```python
from build123d import *

# Parameters (mm, degrees)
BOSS_EXTRUDE1_DEPTH      = 8.255
SKETCH2_R                = 4.52165068
CUT_EXTRUDE1_DEPTH       = 24.892
BOSS_EXTRUDE2_DEPTH      = 2.54
BOSS_EXTRUDE2_DEPTH_BACK = 19.05
BOSS_EXTRUDE3_DEPTH      = 55.87439679
SKETCH8_W                = 306.493093546
SKETCH8_H                = 19.05
BOSS_EXTRUDE4_DEPTH      = 55.87439679
SKETCH9_R                = 88.9
BOSS_EXTRUDE5_DEPTH      = 19.05
SKETCH10_W               = 191.766813877
SKETCH10_H               = 13.52799874
BOSS_EXTRUDE6_DEPTH      = 55.87439679
SKETCH12_R               = 1.75
CUT_EXTRUDE3_DEPTH       = 25.146
SKETCH14_R               = 12.700759967
CUT_EXTRUDE4_DEPTH       = 30.48
CUT_EXTRUDE5_DEPTH       = 55.118
SKETCH16_R               = 79.375
CUT_EXTRUDE6_DEPTH       = 16.129
CUT_EXTRUDE7_DEPTH       = 8.89
CUT_EXTRUDE8_DEPTH       = 2.54
SKETCH19_W               = 282.174011185
SKETCH19_H               = 80.01
CUT_EXTRUDE9_DEPTH       = 75.946
SKETCH20_R               = 79.375
BOSS_EXTRUDE7_DEPTH      = 19.05
SKETCH21_R               = 2.8
SKETCH21_R_2             = 2.794
CUT_EXTRUDE10_DEPTH      = 9.1
SKETCH22_R               = 79.375
CUT_EXTRUDE11_DEPTH      = 18.161
BOSS_EXTRUDE8_DEPTH      = 5.08
SKETCH24_R               = 80.01
CUT_EXTRUDE12_DEPTH      = 18.161


with BuildPart() as part:
    # Sketch1 → Boss-Extrude1 (new, symmetric)
    with BuildSketch(Plane(origin=(0, 0, 0), x_dir=(1, 0, 0), z_dir=(0, 1, 0))):
        Polygon((-26.685513069, 19.73834527), (-3.435840979, 33.16154971), (26.859514241, -19.311544765), (3.609842152, -32.734749204), align=None)
    extrude(amount=BOSS_EXTRUDE1_DEPTH, both=True)

    # Sketch2 → Cut-Extrude1 (cut)
    with BuildSketch(Plane(origin=(0, 8.255, 0), x_dir=(1, 0, 0), z_dir=(0, 1, 0))):
        with Locations(Location((0, 0, 0), (0, 0, 270))):
            Circle(SKETCH2_R)
    extrude(amount=-CUT_EXTRUDE1_DEPTH, mode=Mode.SUBTRACT)

    # Sketch12 → Cut-Extrude3 (cut)
    with BuildSketch(Plane(origin=(0, 8.255, 0), x_dir=(1, 0, 0), z_dir=(0, 1, 0))):
        with Locations(Location((-3.182842434, 15.553762143, 0), (0, 0, 270))):
            Circle(SKETCH12_R)
        with Locations(Location((3.182843419, -15.553761764, 0), (0, 0, 270))):
            Circle(SKETCH12_R)
        with Locations(Location((-11.87853102, 10.533303997, 0), (0, 0, 270))):
            Circle(SKETCH12_R)
        with Locations(Location((11.878532006, -10.533303617, 0), (0, 0, 270))):
            Circle(SKETCH12_R)
    extrude(amount=-CUT_EXTRUDE3_DEPTH, mode=Mode.SUBTRACT)


with BuildPart() as body_2:
    # Sketch3 → Boss-Extrude2 (new, two sides: drawn at the far end of the back side and taken through both)
    with BuildSketch(Plane(origin=(0, 8.255, 0), x_dir=(1, 0, 0), z_dir=(0, 1, 0)).offset(-BOSS_EXTRUDE2_DEPTH_BACK)):
        Polygon((-10.314271596, 73.739239236), (-58.702918637, 45.802040841), (10.314271596, -73.739239236), (58.702918637, -45.802040841), align=None)
        Polygon((-26.685513069, 19.73834527), (3.609842152, -32.734749204), (26.859514241, -19.311544765), (-3.435840979, 33.16154971), align=None, mode=Mode.SUBTRACT)
    extrude(amount=BOSS_EXTRUDE2_DEPTH + BOSS_EXTRUDE2_DEPTH_BACK)

    # Sketch7 → Boss-Extrude3 (add)
    with BuildSketch(Plane(origin=(-24.19432352, 0, 13.968599197), x_dir=(0.5000000000000003, 0, 0.8660254037844384), z_dir=(-0.8660254037844385, 0, 0.5000000000000004))):
        Polygon((-90.607190232, 10.795), (-118.92932164, -90.805), (-97.33932164, -90.805), (-69.017190232, -10.795), (-69.017190232, 10.795), align=None)
    boss_extrude3 = extrude(amount=-BOSS_EXTRUDE3_DEPTH)

    # Sketch8 → Boss-Extrude4 (add)
    with BuildSketch(Plane(origin=(-24.19432352, 0, 13.968599197), x_dir=(0.5000000000000003, 0, 0.8660254037844384), z_dir=(-0.8660254037844385, 0, 0.5000000000000004))):
        with Locations((0, -100.33)):
            Rectangle(SKETCH8_W, SKETCH8_H)
    extrude(amount=-BOSS_EXTRUDE4_DEPTH)

    # Mirror1: Boss-Extrude3 across plane
    add(boss_extrude3.mirror(Plane(origin=(-0.070654873, 0, -0.122377831), x_dir=(-0.8660254037844366, 0, 0.5000000000000038), z_dir=(0.5000000000000041, 0, 0.8660254037844364))))

    # Sketch9 → Boss-Extrude5 (add)
    with BuildSketch(Plane(origin=(0, -90.805, 0), x_dir=(1, 0, 0), z_dir=(0, 1, 0))):
        Circle(SKETCH9_R)
    extrude(amount=-BOSS_EXTRUDE5_DEPTH)

    # Sketch10 → Boss-Extrude6 (add)
    with BuildSketch(Plane(origin=(-24.19432352, 0, 13.968599197), x_dir=(0.5000000000000047, 0, 0.866025403784436), z_dir=(-0.866025403784436, 0, 0.5000000000000047))):
        with Locations((-2.1166315, -68.398848488)):
            Rectangle(SKETCH10_W, SKETCH10_H)
    extrude(amount=-BOSS_EXTRUDE6_DEPTH)

    # Sketch14 → Cut-Extrude4 (cut)
    with BuildSketch(Plane(origin=(0, 10.795, 0), x_dir=(1, 0, 0), z_dir=(0, 1, 0))):
        with Locations(Location((24.120133011, -48.16621031, 0), (0, 0, 270))):
            Circle(SKETCH14_R)
    cut_extrude4 = extrude(amount=-CUT_EXTRUDE4_DEPTH, mode=Mode.SUBTRACT)

    # Mirror2: Cut-Extrude4 across plane
    add(cut_extrude4.mirror(Plane(origin=(-0.070654873, 0, -0.122377831), x_dir=(-0.8660254037844366, 0, 0.5000000000000038), z_dir=(0.5000000000000041, 0, 0.8660254037844364))), mode=Mode.SUBTRACT)

    # Sketch15 → Cut-Extrude5 (cut)
    with BuildSketch(Plane(origin=(0, -90.805, 0), x_dir=(1, 0, 0), z_dir=(0, 1, 0))):
        Polygon((100.817596907, -118.746803351), (83.517674594, -88.782458937), (35.129027553, -116.719657331), (52.428949866, -146.684001745), align=None)
        Polygon((-83.658984341, 89.027214598), (-35.2703373, 116.964412993), (-52.428949866, 146.684001745), (-100.817596907, 118.746803351), align=None)
    extrude(amount=-CUT_EXTRUDE5_DEPTH, mode=Mode.SUBTRACT)

    # Sketch16 → Cut-Extrude6 (cut)
    with BuildSketch(Plane(origin=(0, -90.805, 0), x_dir=(1, 0, 0), z_dir=(0, 1, 0))):
        with Locations(Location((0, 0, 0), (0, 0, 270))):
            Circle(SKETCH16_R)
    extrude(amount=-CUT_EXTRUDE6_DEPTH, mode=Mode.SUBTRACT)


with BuildPart() as cut_extrude7_tool:
    # Sketch17 → Cut-Extrude7 (new body)
    with BuildSketch(Plane(origin=(0, 10.795, 0), x_dir=(1, 0, 0), z_dir=(0, 1, 0))):
        Polygon((27.82393906, -104.066872908), (76.212586101, -76.129674513), (-31.017857396, 109.598901741), (-79.406504437, 81.661703346), align=None)
    extrude(amount=-CUT_EXTRUDE7_DEPTH)


with BuildPart() as part_1:
    add(part.part)

    # Cut-Extrude7: cut by cut_extrude7_tool
    add(cut_extrude7_tool.part, mode=Mode.SUBTRACT)

    # Sketch18 → Cut-Extrude8 (cut)
    with BuildSketch(Plane(origin=(0, 1.905, 0), x_dir=(1, 0, 0), z_dir=(0, 1, 0))):
        Polygon((-26.685513069, 19.73834527), (3.609842152, -32.734749204), (26.859514241, -19.311544765), (-3.435840979, 33.16154971), align=None)
    extrude(amount=-CUT_EXTRUDE8_DEPTH, mode=Mode.SUBTRACT)


with BuildPart() as body_2_1:
    add(body_2.part)

    # Cut-Extrude7: cut by cut_extrude7_tool
    add(cut_extrude7_tool.part, mode=Mode.SUBTRACT)

    # Sketch19 → Cut-Extrude9 (cut)
    with BuildSketch(Plane(origin=(-24.19432352, 0, 13.968599197), x_dir=(0.5000000000000047, 0, 0.866025403784436), z_dir=(-0.866025403784436, 0, 0.5000000000000047))):
        with Locations((-0.70763264, -50.8)):
            Rectangle(SKETCH19_W, SKETCH19_H)
    extrude(amount=-CUT_EXTRUDE9_DEPTH, mode=Mode.SUBTRACT)


with BuildPart() as cut_extrude9_piece_1:
    # of the separate pieces the step leaves, piece 1, a body of its own (cut_extrude9_pieces)
    add(body_2_1.part.solids().sort_by_distance((-83.658984341, -90.805, -89.027214598))[0])

    # Sketch20 → Boss-Extrude7 (add)
    with BuildSketch(Plane.XZ.offset(109.855)):
        with BuildLine():
            Line((-83.658984341, -89.027214598), (-35.2703373, -116.964412993))
            ThreePointArc((-35.2703373, -116.964412993), (76.919154391, -44.572464934), (83.517674594, 88.782458937))
            Line((83.517674594, 88.782458937), (35.129027553, 116.719657331))
            ThreePointArc((35.129027553, 116.719657331), (-77.953106839, 44.843076777), (-83.658984341, -89.027214598))
        make_face()
        with Locations(Location((0, 0, 0), (0, 0, 90))):
            Circle(SKETCH20_R, mode=Mode.SUBTRACT)
    extrude(amount=-BOSS_EXTRUDE7_DEPTH)

    # Sketch21 → Cut-Extrude10 (cut)
    with BuildSketch(Plane(origin=(0, -90.805, 0), x_dir=(1, 0, 0), z_dir=(0, 1, 0))):
        with Locations(Location((-10.611856409, 101.680071559, 0), (0, 0, 270))):
            Circle(SKETCH21_R)
        with Locations(Location((-82.751596824, 60.030173011, 0), (0, 0, 270))):
            Circle(SKETCH21_R)
        with Locations(Location((82.610287077, -59.78541735, 0), (0, 0, 270))):
            Circle(SKETCH21_R)
        with Locations(Location((10.470546662, -101.435315897, 0), (0, 0, 270))):
            Circle(SKETCH21_R)
        with Locations(Location((44.477086399, 72.035469588, 0), (0, 0, 270))):
            Circle(SKETCH21_R_2)
        with Locations(Location((86.011031333, 5.793902801, 0), (0, 0, 270))):
            Circle(SKETCH21_R_2)
    extrude(amount=-CUT_EXTRUDE10_DEPTH, mode=Mode.SUBTRACT)

    # Sketch22 → Cut-Extrude11 (cut)
    with BuildSketch(Plane(origin=(0, -90.805, 0), x_dir=(1, 0, 0), z_dir=(0, 1, 0))):
        with Locations(Location((0, 0, 0), (0, 0, 270))):
            Circle(SKETCH22_R)
    extrude(amount=-CUT_EXTRUDE11_DEPTH, mode=Mode.SUBTRACT)

    # Sketch23 → Boss-Extrude8 (add)
    with BuildSketch(Plane.XZ.offset(109.855)):
        with BuildLine():
            Line((-83.658984341, -89.027214598), (-35.2703373, -116.964412993))
            ThreePointArc((-35.2703373, -116.964412993), (76.919154391, -44.572464934), (83.517674594, 88.782458937))
            Line((83.517674594, 88.782458937), (35.129027553, 116.719657331))
            ThreePointArc((35.129027553, 116.719657331), (-77.953106839, 44.843076777), (-83.658984341, -89.027214598))
        make_face()
    extrude(amount=BOSS_EXTRUDE8_DEPTH)

    # Sketch24 → Cut-Extrude12 (cut)
    with BuildSketch(Plane(origin=(0, -90.805, 0), x_dir=(1, 0, 0), z_dir=(0, 1, 0))):
        with Locations((-0.739793922, -0.263949779)):
            Circle(SKETCH24_R)
    extrude(amount=-CUT_EXTRUDE12_DEPTH, mode=Mode.SUBTRACT)


with BuildPart() as cut_extrude9_piece_2:
    # of the separate pieces the step leaves, piece 2, a body of its own (cut_extrude9_pieces)
    add(body_2_1.part.solids().sort_by_distance((-70.737011886, 1.905, -66.645701772))[0])


with BuildPart() as cut_extrude9_piece_2_1:
    # Body-Move/Copy1: moved
    add(cut_extrude9_piece_2.part.moved(Location((0, -38.1, 0))))


with BuildPart() as part_2:
    # Body-Move/Copy1: moved
    add(part_1.part.moved(Location((0, -38.1, 0))))


with BuildPart() as cut_extrude9_piece_2_2:
    add(cut_extrude9_piece_2_1.part)

    # Combine1: union part
    add(part_2.part)


solid = cut_extrude9_piece_1.part
```
Can you work these out from the model? Positions are in its coordinate system, mm. A direction names the side the tool comes from. Give positions to 0.01 mm unless a question says otherwise; leave off trailing zeros. Loops run counter-clockwise (first coordinate to the right, second up) from the corner with the lowest first, then second, coordinate; pieces in that order, holes last. Notation, with made-up numbers: M -32,17.25 L -23,17.25 A21 ccw -23,26.25 Z; hole C 30,72 d2. An arc over 180 degrees is marked long. Answer in a Markdown table with one row per item.
1. Suppose I cut it at C-C on z = -27. Write out the boundary of the cut face in (x, y) (3 decimals), plus the area to 3 significant figures.
Taken from the geometry:
| item | result |
|---|---|
| outline | M -97.352,-114.935 L 85.551,-114.935 L 85.551,-90.805 L 74.642,-90.805 L 74.642,-108.966 L -75.961,-108.966 L -75.961,-90.805 L -97.352,-90.805 Z |
| area | 1,680 mm² |
2. For pin 1 Ø1 at (y, z) = (-112.5, 75.5) entering from -X; pin 2 Ø1.5 at (y, z) = (-95, 56) entering from +X; pin 3 Ø5 at (x, z) = (21, 28.5) entering from +Y, each with a flat end and sliding along its axis, tell me the tip position at first contact or that it passes through.
Taken from the geometry:
| item | result |
|---|---|
| pin 1 | stops at x = -54.77 |
| pin 2 | stops at x = 94.05 |
| pin 3 | stops at y = -108.97 |
3. If I drill on line 1 along Y through (x, z) = (25, -21.5) (3 decimals); line 2 along Z through (x, y) = (-35, -100.25); line 3 along Z through (x, y) = (-43.5, -102), over which ranges is the centre line in solid material (lowest first)?
Taken from the geometry:
| item | result |
|---|---|
| line 1 | y = -114.935 to -108.966 |
| line 2 | z = -116.94 to -72.04, 72.57 to 91.48 |
| line 3 | z = -112.21 to -67.36, 67.89 to 85.12 |
4. Which directions (+Z, -Z, +X, -X, +Y, -Y) give clear straight access to the entire face, cutting with the end or side of a thin tool? Please do faces 1 (the cylindrical face through (75.937, -102.701, -46.247)), 2 (the flat face through (-11, -99.905, -102)).
Taken from the geometry:
| item | result |
|---|---|
| face 1 | +X, +Y, -Y |
| face 2 | +Y |
5. Thinking about a two-plate mould opening in X: for faces 3 (the flat face through (-83, -99.905, -60)), 4 (the flat face through (59.662, -102.701, 102.555)), 5 (the flat face through (-59.8, -102.7, -102.8)), which applies, released by +X, released by -X, zero draft, split by the parting line, or undercut?
Taken from the geometry:
| item | result |
|---|---|
| face 3 | undercut |
| face 4 | released by +X |
| face 5 | released by -X |
6. Suppose I cut it at D-D on z = -84. Write out the boundary of the cut face in (x, y) (1 decimal).
Taken from the geometry:
| item | result |
|---|---|
| outline | M -85.9,-114.9 L 43.6,-114.9 L 43.6,-90.8 L -85.9,-90.8 Z |
7. Suppose I cut it at B-B on x = 59.5. Write out the boundary of the cut face in (y, z) (3 decimals).
Taken from the geometry:
| item | result |
|---|---|
| outline | M -114.935,-68.69 L -90.805,-68.69 L -90.805,-52.537 L -108.966,-52.537 L -108.966,52.921 L -90.805,52.921 L -90.805,102.649 L -114.935,102.649 Z |
